Source: three-view drawing plus pictorial views. Frame: mm from the lowest corner of the part. A direction names the side the tool comes from. Round coordinates to 2 decimals unless told otherwise and drop trailing zeros. Order: outer loops, then holes, each group sorted by start corner. A loop starts at its lowest first (then second) coordinate and runs counter-clockwise, first axis right, second up. Notation, with made-up numbers: (79, 39) -> (122, 39) arc R12 cw to (122, 58) -> close; hole circle Ø10 at (-23.5, 17). An arc over 180 degrees is marked (long way). Use a Markdown table: item, result.
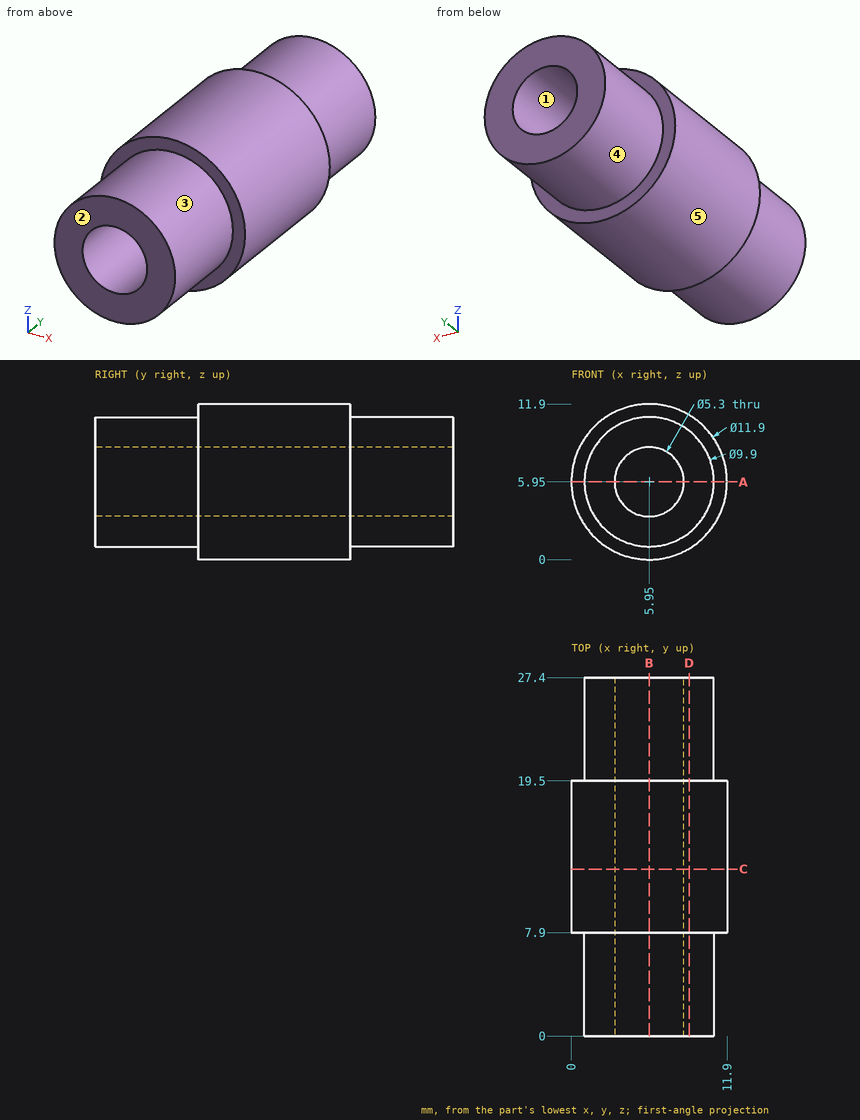
1) Set-up query: the marked faces 4 and 5. Return all of +Z, -Z, +X, -X, +Y, -Y with unobstructed straight access to the full face (end or side cutting, diameter ignored); none if empty.
Results found:
| item | result |
|---|---|
| face 4 | +Y |
| face 5 | +Y, -Y |
2) Cut plane C-C on y = 12.75. Return loops of the section in (x, z).
Results found:
| item | result |
|---|---|
| outline | circle Ø11.9 at (5.95, 5.95); hole circle Ø5.3 at (5.95, 5.95) |
3) Pull-direction query (Z, two-part tool) for the marked faces 1, 2 and 3; classes: +Z half, -Z half, draft (parallel to the pull), parting line (faces both ways), or undercut.
Results found:
| item | result |
|---|---|
| face 1 | undercut |
| face 2 | draft |
| face 3 | parting line |
4) Cut plane B-B on x = 5.95. Return loops of the section in (y, z), and give its area (3 significant figures).
Results found:
| item | result |
|---|---|
| outline | (0, 1) -> (7.9, 1) -> (7.9, 0) -> (19.5, 0) -> (19.5, 1) -> (27.4, 1) -> (27.4, 3.3) -> (0, 3.3) -> close; (0, 8.6) -> (27.4, 8.6) -> (27.4, 10.9) -> (19.5, 10.9) -> (19.5, 11.9) -> (7.9, 11.9) -> (7.9, 10.9) -> (0, 10.9) -> close |
| area | 149 mm² |
5) Cut plane D-D on x = 9. Return loops of the section in (y, z), and give its area (3 significant figures).
Results found:
| item | result |
|---|---|
| outline | (0, 2.05) -> (7.9, 2.05) -> (7.9, 0.84) -> (19.5, 0.84) -> (19.5, 2.05) -> (27.4, 2.05) -> (27.4, 9.85) -> (19.5, 9.85) -> (19.5, 11.06) -> (7.9, 11.06) -> (7.9, 9.85) -> (0, 9.85) -> close |
| area | 242 mm² |
6) Cut plane A-A on z = 5.95. Return loops of the section in (x, y).
Results found:
| item | result |
|---|---|
| outline | (0, 7.9) -> (1, 7.9) -> (1, 0) -> (3.3, 0) -> (3.3, 27.4) -> (1, 27.4) -> (1, 19.5) -> (0, 19.5) -> close; (8.6, 0) -> (10.9, 0) -> (10.9, 7.9) -> (11.9, 7.9) -> (11.9, 19.5) -> (10.9, 19.5) -> (10.9, 27.4) -> (8.6, 27.4) -> close |
7) Line query: L1, parallel to Z at x = 5.95, y = 15.5; L2, parallel to Y at x = 9, z = 11; L3, parallel to X at y = 13.25, z = 7. Output: solid intervals per line, ascending. Write a range as [from, to].
Results found:
| item | result |
|---|---|
| L1 | z = [0, 3.3], [8.6, 11.9] |
| L2 | y = [7.9, 19.5] |
| L3 | x = [0.09, 3.52], [8.38, 11.81] |
8) Pin query (flat end, axial travel): pin 1 Ø7 at (x, z) = (5.95, 5.95) entering from -Y; pin 2 Ø1.5 at (y, z) = (24, 10) entering from +X. Return the tip coordinate at first contact, or that it passes through.
Results found:
| item | result |
|---|---|
| pin 1 | stops at y = 0 |
| pin 2 | stops at x = 9.64 |
